Can you work these out from the drawing? Everything is in mm from the part's minimum corner. A direction names the side the tool comes from. Round coordinates to 2 decimals unless told otherwise and drop trailing zeros. Order: outer loops, then holes, each group sorted by start corner. A loop starts at its lowest first (then second) coordinate and runs counter-clockwise, first axis right, second up. Notation, with made-up numbers: (-26.75, 14.5) - (24.25, 14.5) arc R8 ccw to (24.25, 24.5) - close; hole circle Ø11 at (-9.5, 82.5). An arc over 180 degrees is marked (long way). Write item = value, one per line.
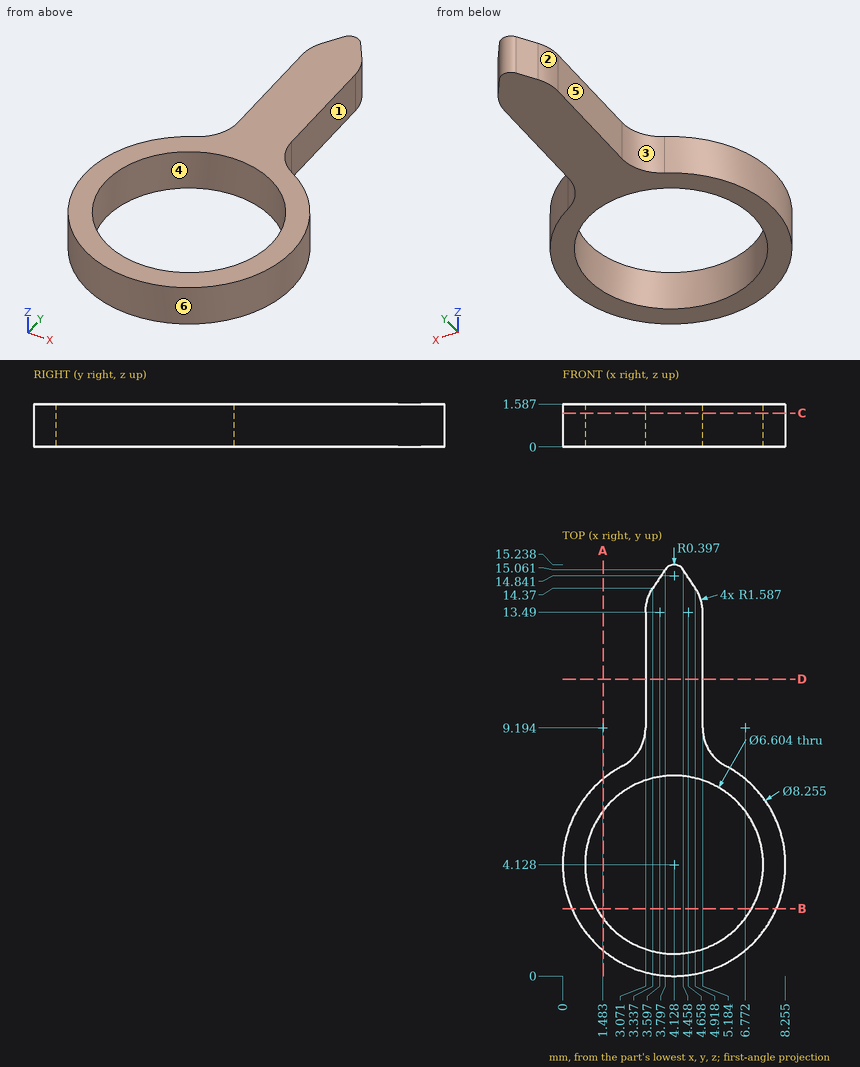
(1) Thinking about a two-plate mould opening in Y: for the marked faces 3, 4, 5 and 6, which applies, +Y half, -Y half, draft (parallel to the pull), parting line (faces both ways), or undercut?
Computed:
face_3 = +Y half
face_4 = undercut
face_5 = draft
face_6 = parting line
(2) If we section it at D-D (y = 11): Write out the boundary of the cut face in (x, z) (1 decimal).
Computed:
outline = (3.1, 0) - (5.2, 0) - (5.2, 1.6) - (3.1, 1.6) - close
(3) If we section it at B-B (y = 2.5): Write out the boundary of the cut face in (x, z) (1 decimal).
Computed:
outline = (0.3, 0) - (1.3, 0) - (1.3, 1.6) - (0.3, 1.6) - close; (7, 0) - (7.9, 0) - (7.9, 1.6) - (7, 1.6) - close
(4) Will these pins go through, and if not, where does the flat tip stop? P1, Ø0.5, axis at y = 12.5, z = 1, coming from the -X side; P2, Ø1, axis at x = 6, y = 5.5, coming from the -Z side.
Computed:
P1 = 3.07
P2 = through
(5) If we section it at C-C (z = 1.25): Write out the boundary of the cut face in (x, y) (1 decimal).
Computed:
outline = (2.2, 7.8) arc R4.1 ccw (long way) to (6, 7.8) arc R1.6 cw to (5.2, 9.2) - (5.2, 13.5) arc R1.6 ccw to (4.9, 14.4) - (4.5, 15.1) arc R0.4 ccw to (3.8, 15.1) - (3.3, 14.4) arc R1.6 ccw to (3.1, 13.5) - (3.1, 9.2) arc R1.6 cw to start; hole circle Ø6.6 at (4.1, 4.1)
(6) If we section it at A-A (x = 1.5): Write out the boundary of the cut face in (y, z) (1 decimal).
Computed:
outline = (0.9, 0) - (2.1, 0) - (2.1, 1.6) - (0.9, 1.6) - close; (6.1, 0) - (7.3, 0) - (7.3, 1.6) - (6.1, 1.6) - close
(7) On a 3-axis mill with a long thin cutter (end or side, diameter ignored), from which of +Z, -Z, +X, -X, +Y, -Y can I reach the whole of each face in a straight line? I mean the marked faces 1 and 2. Say none if no direction works.
Computed:
face_1 = +Z, -Z, +X, +Y
face_2 = +Z, -Z, -X, +Y
(8) If I drill on line 1 (X direction, y = 4.25, z = 1.4); line 2 (X direction, y = 12.75, z = 0.75) (1 decimal); line 3 (X direction, y = 1.5, z = 1.3) (1 decimal), over which ranges is the centre line in solid material (lowest first)? Write a range as from..to.
Computed:
line_1 = 0..0.83, 7.43..8.25
line_2 = 3.1..5.2
line_3 = 0.9..2.1, 6.1..7.3
